Could you check a few things on this model? Use its own coordinates, in mm. Coordinates: 2 decimals unless noted, no trailing zeros. Order: outer loops, then holes, each group sorted by start corner. A loop starts at its lowest first (then second) coordinate and runs counter-clockwise, first axis right, second up. Notation, with made-up numbers: (46.25, -21.5) -> (105.25, -21.5) arc R31 cw to (105.25, 4.5) -> close; hole circle Ø6 at (74, 75.5). An arc over 180 degrees is marked (long way). Use a Markdown table: item, result. Add a question column.
1) If we section it at A-A (y = -57.5): Write out the boundary of the cut face in (x, z) (3 decimals).
2) If we section it at B-B (x = -97): Write out the boundary of the cut face in (y, z) (3 decimals).
3) Will these pins go through, and if not, where does the flat tip stop? pin 1 Ø2 at (x, y) = (-56, 66.5) entering from +Z; pin 2 Ø1.5 at (x, z) = (-67, -2) entering from +Y.
4) If I drill on L1, parallel to Y at x = 13.5, z = -1.8; L2, parallel to Y at x = -52, z = -0.75; L3, parallel to Y at x = 52.5, z = -2, over which ranges is the centre line in solid material (lowest first)? Write a range as [from, to].
```python
from build123d import *

# Parameters (mm, degrees)
FLANGE_BASE1_DEPTH               = 3.175
ESBO_O6_R                        = 1.65
CORTE_EXTRUS_O1_DEPTH            = 10
ESBO_O8_R                        = 11.3
ESBO_O8_R_2                      = 1.65
CORTE_EXTRUS_O3_DEPTH            = 10
PADR_OCIRCULAR1_COUNT            = 4
ESBO_O7_R                        = 1.75
CORTE_EXTRUS_O2_DEPTH            = 10
CHANFRO1_SIZE                    = 2
PADR_OCIRCULAR2_COUNT            = 6
CHANFRO1_OF_PADR_OCIRCULAR2_SIZE = 2
ESPELHAR1_COPY_1_SKETCH_R        = 11.3
ESPELHAR1_COPY_1_SKETCH_R_2      = 1.65
ESPELHAR1_COPY_1_DEPTH           = 10
ESPELHAR1_COPY_2_SKETCH_R        = 11.3
ESPELHAR1_COPY_2_SKETCH_R_2      = 1.65
ESPELHAR1_COPY_2_DEPTH           = 10
ESPELHAR1_COPY_3_SKETCH_R        = 11.3
ESPELHAR1_COPY_3_SKETCH_R_2      = 1.65
ESPELHAR1_COPY_3_DEPTH           = 10
ESBO_O11_R                       = 2.5
CORTE_EXTRUS_O5_DEPTH            = 10
ESBO_O12_R                       = 1.65
CORTE_EXTRUS_O6_DEPTH            = 10
ESBO_O13_W                       = 376.359651272
ESBO_O13_H                       = 358.929615965
CORTE_EXTRUS_O7_DEPTH            = 10
CAVIDADE1_START                  = -5
CAVIDADE1_DEPTH                  = 10


# Read off the part's stored shape, not the designer's step: Cavidade1
# Sheet-metal steps are written as plain solids
with BuildPart() as part:
    # Esboço1 → Flange-base1 (new body)
    with BuildSketch(Plane.XY):
        Polygon((63.508529611, 110), (127.017059222, 0), (63.508529611, -110), (-63.508529611, -110), (-127.017059222, 0), (-63.508529611, 110), align=None)
        Polygon((61, 31.176914536), (-61, 31.176914536), (-79, 0), (-55.905989232, -40), (55.905989232, -40), (79, 0), align=None, mode=Mode.SUBTRACT)
    extrude(amount=-FLANGE_BASE1_DEPTH)

    # Esboço6 → Corte-extrusão1 (cut)
    with BuildSketch(Plane.XY):
        with BuildLine():
            Line((15.65, -73), (-15.65, -73))
            ThreePointArc((-15.65, -73), (-20.316904756, -71.066904756), (-22.25, -66.4))
            Line((-22.25, -66.4), (-22.25, -54.6))
            ThreePointArc((-22.25, -54.6), (-20.316904756, -49.933095244), (-15.65, -48))
            Line((-15.65, -48), (15.65, -48))
            ThreePointArc((15.65, -48), (20.316904756, -49.933095244), (22.25, -54.6))
            Line((22.25, -54.6), (22.25, -66.4))
            ThreePointArc((22.25, -66.4), (20.316904756, -71.066904756), (15.65, -73))
        make_face()
        with Locations((-23.7, -49.9)):
            Circle(ESBO_O6_R)
        with Locations((23.7, -49.9)):
            Circle(ESBO_O6_R)
        with Locations((25.2, -68)):
            Circle(ESBO_O6_R)
        with Locations((-25.2, -68)):
            Circle(ESBO_O6_R)
    extrude(amount=-CORTE_EXTRUS_O1_DEPTH, mode=Mode.SUBTRACT)

    # Esboço8 → Corte-extrusão3 (cut)
    with BuildSketch(Plane.XY):
        with Locations((-33, 60.0982)):
            Circle(ESBO_O8_R)
        with Locations((-20.75, 47.8482)):
            Circle(ESBO_O8_R_2)
    corte_extrus_o3 = extrude(amount=-CORTE_EXTRUS_O3_DEPTH, mode=Mode.SUBTRACT)

    # PadrãoCircular1: Corte-extrusão3 ×4 about axis
    padr_ocircular1_axis = Axis((-33, 60.0982, 0), (0, 0, 1))
    for i in range(1, PADR_OCIRCULAR1_COUNT):
        add(corte_extrus_o3.rotate(padr_ocircular1_axis, i * 360 / PADR_OCIRCULAR1_COUNT), mode=Mode.SUBTRACT)

    # Esboço7 → Corte-extrusão2 (cut)
    with BuildSketch(Plane.XY):
        with Locations((-30, -83)):
            Circle(ESBO_O7_R)
        with Locations((30, -83)):
            Circle(ESBO_O7_R)
    corte_extrus_o2 = extrude(amount=-CORTE_EXTRUS_O2_DEPTH, mode=Mode.SUBTRACT)

    # Chanfro1
    chanfro1_edges = [part.edges().sort_by_distance(p)[0] for p in [
        (-31.75, -83, 0),
        (28.25, -83, 0),
    ]]
    chamfer(chanfro1_edges, length=CHANFRO1_SIZE)

    # PadrãoCircular2: Corte-extrusão2 ×6 about axis
    padr_ocircular2_axis = Axis((0, 0, 0), (0, 0, 1))
    for i in range(1, PADR_OCIRCULAR2_COUNT):
        add(corte_extrus_o2.rotate(padr_ocircular2_axis, i * 360 / PADR_OCIRCULAR2_COUNT), mode=Mode.SUBTRACT)

    # Chanfro1 of PadrãoCircular2
    chanfro1_of_padr_ocircular2_edges = [part.edges().sort_by_distance(p)[0] for p in [
        (56.005108514, -68.99630657, 0),
        (86.005108514, -17.034782343, 0),
        (87.755108514, 14.00369343, 0),
        (57.755108514, 65.965217657, 0),
        (31.75, 83, 0),
        (-28.25, 83, 0),
        (-56.005108514, 68.99630657, 0),
        (-86.005108514, 17.034782343, 0),
        (-87.755108514, -14.00369343, 0),
        (-57.755108514, -65.965217657, 0),
    ]]
    chamfer(chanfro1_of_padr_ocircular2_edges, length=CHANFRO1_OF_PADR_OCIRCULAR2_SIZE)

    # Espelhar1: Corte-extrusão3 across plane
    add(corte_extrus_o3.mirror(Plane(origin=(0, 0, 0), x_dir=(0, 0, 1), z_dir=(1, 0, 0))), mode=Mode.SUBTRACT)

    # Espelhar1 copy 1 sketch → Espelhar1 copy 1 (cut)
    with BuildSketch(Plane(origin=(-27.0982, 93.0982, 0), x_dir=(0, 1, 0), z_dir=(0, 0, 1))):
        with Locations((-33, -60.0982)):
            Circle(ESPELHAR1_COPY_1_SKETCH_R)
        with Locations((-20.75, -47.8482)):
            Circle(ESPELHAR1_COPY_1_SKETCH_R_2)
    extrude(amount=-ESPELHAR1_COPY_1_DEPTH, mode=Mode.SUBTRACT)

    # Espelhar1 copy 2 sketch → Espelhar1 copy 2 (cut)
    with BuildSketch(Plane(origin=(66, 120.1964, 0), x_dir=(1, 0, 0), z_dir=(0, 0, 1))):
        with Locations((-33, -60.0982)):
            Circle(ESPELHAR1_COPY_2_SKETCH_R)
        with Locations((-20.75, -47.8482)):
            Circle(ESPELHAR1_COPY_2_SKETCH_R_2)
    extrude(amount=-ESPELHAR1_COPY_2_DEPTH, mode=Mode.SUBTRACT)

    # Espelhar1 copy 3 sketch → Espelhar1 copy 3 (cut)
    with BuildSketch(Plane(origin=(93.0982, 27.0982, 0), x_dir=(0, -1, 0), z_dir=(0, 0, 1))):
        with Locations((-33, -60.0982)):
            Circle(ESPELHAR1_COPY_3_SKETCH_R)
        with Locations((-20.75, -47.8482)):
            Circle(ESPELHAR1_COPY_3_SKETCH_R_2)
    extrude(amount=-ESPELHAR1_COPY_3_DEPTH, mode=Mode.SUBTRACT)

    # Esboço11 → Corte-extrusão5 (cut)
    with BuildSketch(Plane(origin=(0, 0, -3.175), x_dir=(-1, 0, 0), z_dir=(0, 0, -1))):
        with Locations((-52.5, 90.932667397)):
            Circle(ESBO_O11_R)
        with Locations((-105, 0)):
            Circle(ESBO_O11_R)
        with Locations((52.5, 90.932667397)):
            Circle(ESBO_O11_R)
        with Locations((105, 0)):
            Circle(ESBO_O11_R)
        with Locations((52.5, -90.932667397)):
            Circle(ESBO_O11_R)
        with Locations((-52.5, -90.932667397)):
            Circle(ESBO_O11_R)
    extrude(amount=-CORTE_EXTRUS_O5_DEPTH, mode=Mode.SUBTRACT)

    # Esboço12 → Corte-extrusão6 (cut)
    with BuildSketch(Plane.XY):
        with Locations((-55.257737945, -44.5259)):
            Circle(ESBO_O12_R)
        with Locations((-82.980762114, -0.195772981)):
            Circle(ESBO_O12_R)
        with Locations((-55.257737945, 35.4741)):
            Circle(ESBO_O12_R)
        with Locations((55.257737945, 35.4741)):
            Circle(ESBO_O12_R)
        with Locations((82.980762114, -0.195772981)):
            Circle(ESBO_O12_R)
        with Locations((55.257737945, -44.5259)):
            Circle(ESBO_O12_R)
    extrude(amount=-CORTE_EXTRUS_O6_DEPTH, mode=Mode.SUBTRACT)

    # Esboço13 → Corte-extrusão7 (cut)
    with BuildSketch(Plane.XY):
        with Locations((17.92855311, -8.326549872)):
            Rectangle(ESBO_O13_W, ESBO_O13_H)
        with BuildLine():
            Line((-66.008529611, 105.669872981), (-124.517059222, 4.330127019))
            ThreePointArc((-124.517059222, 4.330127019), (-125.67731326, 0), (-124.517059222, -4.330127019))
            Line((-124.517059222, -4.330127019), (-66.008529611, -105.669872981))
            ThreePointArc((-66.008529611, -105.669872981), (-62.83865663, -108.839745962), (-58.508529611, -110))
            Line((-58.508529611, -110), (58.508529611, -110))
            ThreePointArc((58.508529611, -110), (62.83865663, -108.839745962), (66.008529611, -105.669872981))
            Line((66.008529611, -105.669872981), (124.517059222, -4.330127019))
            ThreePointArc((124.517059222, -4.330127019), (125.67731326, 0), (124.517059222, 4.330127019))
            Line((124.517059222, 4.330127019), (66.008529611, 105.669872981))
            ThreePointArc((66.008529611, 105.669872981), (62.83865663, 108.839745962), (58.508529611, 110))
            Line((58.508529611, 110), (-58.508529611, 110))
            ThreePointArc((-58.508529611, 110), (-62.83865663, 108.839745962), (-66.008529611, 105.669872981))
        make_face(mode=Mode.SUBTRACT)
    extrude(amount=-CORTE_EXTRUS_O7_DEPTH, mode=Mode.SUBTRACT)

    # Cavidade1 outline → Cavidade1 (cut)
    with BuildSketch(Plane.YZ.offset(CAVIDADE1_START)):
        Polygon((-45.825, -3.175), (-48, -1), (-48, -3.175), align=None)
    extrude(amount=CAVIDADE1_DEPTH, mode=Mode.SUBTRACT)


solid = part.part
```
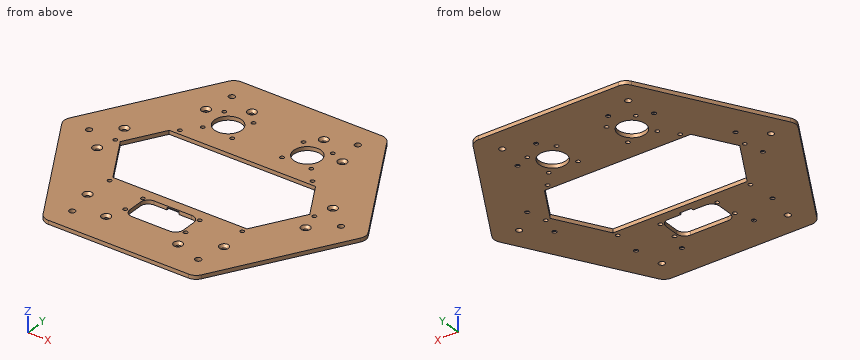
Answer sheet:
| question | item | result |
|---|---|---|
| 1 | outline | (-93.819, -3.175) -> (-22.25, -3.175) -> (-22.25, 0) -> (-93.819, 0) -> close; (22.25, -3.175) -> (93.819, -3.175) -> (93.819, 0) -> (22.25, 0) -> close |
| 2 | outline | (-51.991, -3.175) -> (51.991, -3.175) -> (51.991, 0) -> (-51.991, 0) -> close |
| 3 | pin 1 | z = -1.43 |
| 3 | pin 2 | y = 105.25 |
| 4 | L1 | [-110, -73], [-48, -40], [31.18, 110] |
| 4 | L2 | [-110, -93.38], [-88.48, -40], [31.18, 88.48], [93.38, 110] |
| 4 | L3 | [-110, -93.43], [-88.43, -40], [31.18, 88.43], [93.43, 110] |
